Autodesk Inventor part; units mm, degrees
ref_plane "YZ Plane" through (0, 0, 0) normal (1, 0, 0) x (0, 1, 0)
ref_plane "XZ Plane" through (0, 0, 0) normal (0, 1, 0) x (-1, 0, 0)
ref_plane "XY Plane" through (0, 0, 0) normal (0, 0, 1) x (1, 0, 0)
sketch "Esquisse1" plane through (0, 0, 0) normal (0, 1, 0) x (-1, 0, 0)
  arc A0 (8.3897, -168.8053) -> (8.3897, 132.3637) centre (-777.3166, -18.2208) ccw
  arc A1 (11.3897, -168.8053) -> (11.3897, 132.3637) centre (-774.3166, -18.2208) ccw
  line L0 (11.3897, 132.3637) -> (8.3897, 132.3637)
  line L1 (11.3897, -168.8053) -> (8.3897, -168.8053)
  point P0 (0, 0)
  dimension "d0" = 301.169
extrude "Extrusion1" add sketch "Esquisse1" along normal blind 65
sketch "Esquisse2" plane through (-11.3897, 0, 132.3637) normal (0, 0, 1) x (1, 0, 0)
  line L0 (0, 65) -> (3, 65)
  line L1 (0, 0) -> (3, 0)
  line L2 (0, 65) -> (3, 65)
  line L3 (3, 65) -> (3, 0)
  line L4 (3, 0) -> (0, 0)
  line L5 (0, 0) -> (0, 65)
  point P0 (11.3897, 0)
extrude "Extrusion2" add sketch "Esquisse2" along normal blind 10
sketch "Esquisse3" plane through (-8.3897, 0, -168.8053) normal (0, 0, -1) x (-1, 0, 0)
  line L0 (0, 0) -> (3, 0)
  line L1 (3, 0) -> (3, 65)
  line L2 (0, 0) -> (3, 0)
  line L3 (3, 0) -> (3, 65)
  line L4 (3, 65) -> (0, 65)
  line L5 (0, 65) -> (0, 0)
  point P0 (-8.3897, 0)
extrude "Extrusion3" add sketch "Esquisse3" along normal blind 10
sketch "Esquisse4" plane through (-8.3897, 0, 132.3637) normal (1, 0, 0) x (0, 0, -1)
  line L0 (0, 65) -> (-10, 65)
  line L1 (-10, 65) -> (-8, 65)
  line L2 (-8, 65) -> (-8, 0)
  line L3 (-8, 0) -> (-10, 0)
  line L4 (-10, 0) -> (-10, 65)
  line L5 (301.169, 0) -> (311.169, 0)
  line L6 (301.169, 65) -> (311.169, 65)
  line L7 (311.169, 0) -> (309.169, 0)
  line L8 (309.169, 0) -> (309.169, 65)
  line L9 (309.169, 65) -> (311.169, 65)
  line L10 (311.169, 65) -> (311.169, 0)
  point P0 (132.3637, 0)
  point P1 (309.169, 0)
  dimension "d10" = 2
  dimension "d11" = 2
extrude "Extrusion4" add sketch "Esquisse4" along normal blind 100
sketch "Esquisse5" plane through (0, 0, 0) normal (0, -1, 0) x (1, 0, 0)
  line L0 (91.6103, 140.3637) -> (91.6103, 142.3637)
  line L1 (-11.3897, 142.3637) -> (91.6103, 142.3637)
  line L2 (91.6103, 142.3637) -> (-11.3897, 142.3637)
  line L3 (-11.3897, 132.3637) -> (-11.3897, 142.3637)
  line L4 (-11.3897, 142.3637) -> (-11.3897, 132.3637)
  line L5 (91.6103, -176.8053) -> (91.6103, -178.8053)
  line L6 (91.6103, 142.3637) -> (91.6103, -178.8053)
  line L7 (-11.3897, -178.8053) -> (91.6103, -178.8053)
  line L8 (91.6103, -178.8053) -> (-11.3897, -178.8053)
  line L9 (-11.3897, -168.8053) -> (-11.3897, -178.8053)
  line L10 (-11.3897, -178.8053) -> (-11.3897, -168.8053)
  arc A0 (-11.3897, 132.3637) -> (-11.3897, -168.8053) centre (774.3166, -18.2208) ccw
  point P0 (0, 0)
extrude "Extrusion5" add sketch "Esquisse5" along normal blind 2
sketch "Esquisse7" plane through (91.6103, 0, 132.3637) normal (1, 0, 0) x (0, 0, -1)
  line L0 (301.169, -2) -> (311.169, -2)
  line L1 (-10, 65) -> (311.169, 65)
  line L2 (311.169, 65) -> (311.169, -2)
  line L3 (311.169, -2) -> (-10, -2)
  line L4 (-10, -2) -> (-10, 65)
  point P0 (132.3637, 0)
extrude "Extrusion6" add sketch "Esquisse7" along normal blind 2
sketch "Esquisse8" plane through (-11.3897, 65, -178.8053) normal (-1, 0, 0) x (0, 0, 1)
  line L0 (0, 0) -> (0, -67)
  line L1 (321.169, -67) -> (0, -67)
  line L2 (0, -65) -> (321.169, -65)
  line L3 (321.169, -65) -> (321.169, -67)
  line L4 (321.169, -67) -> (0, -67)
  line L5 (0, -67) -> (0, -65)
  point P0 (178.8053, -65)
extrude "Extrusion7" add sketch "Esquisse8" along normal blind 30
sketch "Esquisse9" plane through (-11.3897, 0, -168.8053) normal (0, 1, 0) x (1, 0, 0)
  arc A0 (0, 0) -> (0, -301.169) centre (785.7064, -150.5845) ccw
  line L0 (0, 0) -> (0, -301.169)
  line L1 (-30, -311.169) -> (-30, 10)
  arc A1 (-15.7, 0) -> (-15.7, -301.169) centre (770.0064, -150.5845) ccw
  line L2 (-15.7, 0) -> (0, 0)
  line L3 (-15.7, -301.169) -> (0, -301.169)
  line L4 (0, -301.169) -> (0, -311.169)
  arc A2 (0, 0) -> (0, -301.169) centre (785.7064, -150.5845) ccw
  line L5 (0, 0) -> (0, 10)
  line L6 (0, 0) -> (0, 10)
  line L7 (-30, 10) -> (-30, -311.169)
  line L8 (0, 10) -> (-30, 10)
  line L9 (-30, 10) -> (-30, -311.169)
  line L10 (0, -311.169) -> (-30, -311.169)
  line L11 (0, -311.169) -> (0, -301.169)
  point P0 (11.3897, -168.8053)
  point P1 (-30, -150.5845)
extrude "Extrusion8" cut sketch "Esquisse9" against normal through all contours L2 A1 L1 L8 L5 | L4 L10 L1 A1 L3
sketch "Esquisse10" plane through (93.6103, 0, 132.3637) normal (1, 0, 0) x (0, 0, -1)
  circle A0 centre (151.5428, 32.5) radius 20
  line L0 (311.169, 65) -> (-10, 65)
  point P0 (132.3637, 0)
  dimension "d36" = 40
  dimension "d37" = 32.5
extrude "Extrusion9" cut sketch "Esquisse10" against normal blind 10
sketch "Esquisse11" plane through (-11.3897, 65, -178.8053) normal (-1, 0, 0) x (0, 0, 1)
  line L0 (10, -65) -> (10, 0)
  line L1 (10, 0) -> (-34.2459, 0)
  line L2 (-34.2459, 0) -> (-34.2459, -126.8111)
  line L3 (-34.2459, -126.8111) -> (10, -126.8111)
  line L4 (10, -126.8111) -> (10, 0)
  line L5 (311.169, -65) -> (311.169, 0)
  line L6 (311.169, 0) -> (416.0548, 0)
  line L7 (416.0548, 0) -> (416.0548, -178.3642)
  line L8 (416.0548, -178.3642) -> (311.169, -178.3642)
  line L9 (311.169, -178.3642) -> (311.169, 0)
  point P0 (178.8053, -65)
extrude "Extrusion10" cut sketch "Esquisse11" against normal through all
sketch "Esquisse12" plane through (91.6103, 0, 132.3637) normal (-1, 0, 0) x (0, 0, 1)
  line L0 (-301.169, 0) -> (0, 0)
  line L1 (-301.169, 65) -> (0, 65)
  line L2 (-301.169, 0) -> (-299.169, 0)
  line L3 (-299.169, 0) -> (-299.169, 65)
  line L4 (-299.169, 65) -> (-301.169, 65)
  line L5 (-301.169, 65) -> (-301.169, 0)
  line L6 (0, 0) -> (-2, 0)
  line L7 (-2, 0) -> (-2, 65)
  line L8 (-2, 65) -> (0, 65)
  line L9 (0, 65) -> (0, 0)
  point P0 (-132.3637, 0)
  point P1 (-2, 0)
  dimension "d42" = 2
  dimension "d43" = 2
extrude "Extrusion11" add sketch "Esquisse12" along normal up to surface contours L5 L1 L3 L0 | L7 L1 L9 L0
properties part number "pièce_fixe_station"
Geometry: final body of the model. Coordinates: model frame, mm. A direction names the side the tool comes from. Round coordinates to 2 decimals unless told otherwise and drop trailing zeros. Loops run counter-clockwise (first coordinate to the right, second up) from the corner with the lowest first, then second, coordinate; pieces in that order, holes last. Notation, with made-up numbers: (31, -27.5) -> (70, -27.5) arc R15 ccw to (70, -11.5) -> close; hole circle Ø8 at (76, 18). An arc over 180 degrees is marked (long way). Use one line per item in the form item = value. Start each with the question number.
1) First-contact query: P1, Ø1, axis at x = 53.5, z = 15.5, coming from the +Y side; P2, Ø8, axis at y = 7.5, z = 9, coming from the -X side. Flat tips, straight axial feed; report the tip coordinate or a pass-through.
2) Section A-A on z = -7. Output: boundary loops of the cut face in (x, y), then the cut area to 3 significant figures.
3) Section C-C on x = 43.5. Output: boundary loops of the cut face in (y, z).
4) Section D-D on y = 32.5. Output: boundary loops of the cut face in (x, z), then the cut area to 3 significant figures.
5) Draft query along X for faces 5 (the cylindrical face through (-41.387, -0.986, -20.342)), 6 (the flat face through (42, 32, -166.805)), 7 (the flat face through (32, 31, -168.805)). Return one class per face: released by +X, released by -X, zero draft, split by the parting line, or undercut.
6) Section B-B on y = 9. Output: boundary loops of the cut face in (x, z).
7) Line query: L1, parallel to Z at x = 80, y = 49.5; L2, parallel to X at y = 59, z = -24; L3, parallel to Z at x = 92, y = 32. Output: solid intervals per line, ascending.
8) Access query for faces 1 (the cylindrical face through (-25.687, 32.955, -20.342)), 2 (the cylindrical face through (92.624, 49.364, -29.931)), 3 (the flat face through (-24, 65, -18)), 4 (the flat face through (42, 32, 130.364)). Directions: +Z, -Z, +X, -X, +Y, -Y. A direction counts if a zero-diameter tool reaches every point of the face in a straight line with its end or side. Return the directions, or none.
Response:
q1.P1 = 0
q1.P2 = -25.35
q2.outline = (-41.31, -2) -> (93.61, -2) -> (93.61, 16.64) -> (91.61, 16.64) -> (91.61, 0) -> (-22.61, 0) -> (-22.61, 65) -> (-25.61, 65) -> (-25.61, 0) -> (-41.31, 0) -> close; (91.61, 48.36) -> (93.61, 48.36) -> (93.61, 65) -> (91.61, 65) -> close
q2.area = 531 mm^2
q3.outline = (-2, -168.81) -> (65, -168.81) -> (65, -166.81) -> (0, -166.81) -> (0, 130.36) -> (65, 130.36) -> (65, 132.36) -> (-2, 132.36) -> close
q4.outline = (-11.39, -168.81) -> (93.61, -168.81) -> (93.61, -39.18) -> (91.61, -39.18) -> (91.61, -166.81) -> (-8.77, -166.81) arc R800.01 cw to (-8.77, 130.36) -> (91.61, 130.36) -> (91.61, 0.82) -> (93.61, 0.82) -> (93.61, 132.36) -> (-11.39, 132.36) arc R800.01 ccw to start
q4.area = 1,830 mm^2
q5.face_5 = released by -X
q5.face_6 = undercut
q5.face_7 = zero draft
q6.outline = (-11.39, -168.81) -> (93.61, -168.81) -> (93.61, 132.36) -> (-11.39, 132.36) arc R800.01 ccw to start; hole (-8.77, -166.81) -> (91.61, -166.81) -> (91.61, 130.36) -> (-8.77, 130.36) arc R800.01 ccw to start
q7.L1 = -168.81 to -166.81, 130.36 to 132.36
q7.L2 = -25.67 to -22.67, 91.61 to 93.61
q7.L3 = -168.81 to -39.17, 0.81 to 132.36
q8.face_1 = -X, +Y
q8.face_2 = +X
q8.face_3 = +Z, -Z, +X, -X, +Y
q8.face_4 = +Y
